CAD build for the part. Positions are in the model's coordinates, mm. Face numbers are marked on the shaded views. A direction names the side the tool comes from. Coordinates: 2 decimals unless noted, no trailing zeros. Loops run counter-clockwise (first coordinate to the right, second up) from the corner with the lowest first, then second, coordinate; pieces in that order, holes last. Notation, with made-up numbers: (31.25, 58.5) -> (59.25, 58.5) arc R22 cw to (59.25, 67.5) -> close; hole circle Ø4 at (-12, 54). An arc over 180 degrees is marked (long way). Return JSON: item names as keys, results as strings. Group by question number.
(1) Tool access for the marked faces 1, 2, 3, 4 and 5: list every direction of +Z, -Z, +X, -X, +Y, -Y with a clear straight run to the whole face (end or side of a thin tool).
(2) Flat gauge pins, fed straight in: pin 1 Ø2.5 at (x, y) = (16.5, 3.5) entering from -Z; pin 2 Ø1.8 at (x, z) = (-16, 17.5) entering from +Y; pin 3 Ø1.5 at (x, z) = (10.5, 27.5) entering from +Y; pin 4 Ø8 at (x, z) = (-12.5, 20.5) entering from +Y. Where does each tip first touch, or does it go through?
(3) Saw through at A-A on x = -1. Write the cut outline in (y, z), then the cut area to 3 significant figures.
(4) Probe L1, parallel to X at y = 5, z = 9.5; L2, parallel to X at y = -1.5, z = 29.5; L3, parallel to Y at x = -1.5, z = 15. List the from-to ranges inside material, lowest first.
(5) Saw through at B-B on y = 2.25. Write the cut outline in (x, z), then the cut area to 3 significant figures.
(6) Mould opens along Z. For the marked faces 6, 7 and 8 say: pulls with the +Z half, pulls with the -Z half, needs draft (parallel to the pull), parting line crosses it, or undercut.
(7) Saw through at C-C on z = 0.5. Write the cut outline in (x, y), then the cut area to 3 significant figures.
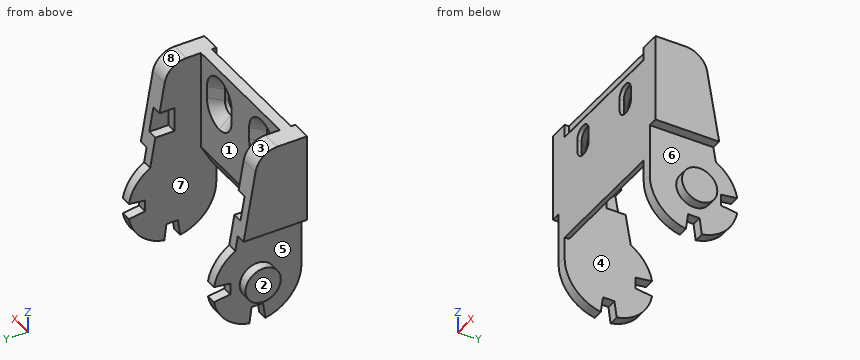
```python
from build123d import *

# Parameters (mm, degrees)
BODY_DEPTH                                       = 32
BODY_DEPTH_BACK                                  = 15
PIVOT_START                                      = 15
PIVOT_PIN_R_SKETCH_R                             = 4
PIVOT_PIN_R_DEPTH                                = 4.25
OUTSIDE_SHAPE_CUT_OUT_DEPTH                      = 40.272286666
OUTSIDE_SHAPE_CUT_OUT_DEPTH_BACK                 = 40.272286666
OUTSIDE_SHAPE_CUT_OUT_SKETCH_W                   = 49
OUTSIDE_SHAPE_CUT_OUT_SKETCH_H                   = 22
OUTSIDE_START                                    = 17.3
OUTSIDE_SHAPE_CUT_OUT_SKETCH_R_W                 = 24
OUTSIDE_SHAPE_CUT_OUT_SKETCH_R_H                 = 24
OUTSIDE_SHAPE_CUT_OUT_SKETCH_R_R                 = 4
OUTSIDE_SHAPE_CUT_OUT_R_DEPTH                    = 22.923727913
INSIDE_START                                     = 15
INSIDE_SHAPE_CUT_OUT_DEPTH                       = 30
LIGHTENING_START                                 = 1.25
LIGHTENING_2_SKETCH_W                            = 34.6
LIGHTENING_2_SKETCH_H                            = 5.5
LIGHTENING_2_DEPTH                               = 38.973727913
F_2_START                                        = -8.25
F_2_LATERAL_SLOTS_ORIENTATED_LONGITUDINALL_DEPTH = 3.5


with BuildPart() as part:
    # Profile Sketch → Body (new, two sides: drawn at the far end of the back side and taken through both)
    with BuildSketch(Plane.XY.offset(-BODY_DEPTH_BACK)):
        Polygon((-19.5, -8.25), (19.5, -8.25), (19.5, 11.75), (15, 11.75), (15, -4.75), (-15, -4.75), (-15, 11.75), (-19.5, 11.75), align=None)
    extrude(amount=BODY_DEPTH + BODY_DEPTH_BACK)

    # Pivot Pin R Sketch → Pivot Pin R (add)
    with BuildSketch(Plane(origin=(0, 0, 0), x_dir=(0, 0, -1), z_dir=(1, 0, 0)).offset(PIVOT_START)):
        with Locations((0, 1.75)):
            Circle(PIVOT_PIN_R_SKETCH_R)
    pivot_pin_r = extrude(amount=PIVOT_PIN_R_DEPTH)

    # Pivot Pin L: Pivot Pin R across plane
    add(pivot_pin_r.mirror(Plane(origin=(0, 0, 0), x_dir=(0, 0, 1), z_dir=(1, 0, 0))))

    # Outside Shape Cut Out Sketch → Outside Shape Cut Out (cut, two sides: drawn at the far end of the back side and taken through both)
    with BuildSketch(Plane(origin=(0, 0, 0), x_dir=(0, 0, -1), z_dir=(1, 0, 0)).offset(-OUTSIDE_SHAPE_CUT_OUT_DEPTH_BACK)):
        with Locations((-9.5, 0.75)):
            Rectangle(OUTSIDE_SHAPE_CUT_OUT_SKETCH_W, OUTSIDE_SHAPE_CUT_OUT_SKETCH_H)
        with BuildLine():
            Line((-27.844593584, 3.462159665), (-8.660254038, 6.75))
            ThreePointArc((-8.660254038, 6.75), (-5.762166553, 9.922969878), (-1.8, 11.586666102))
            Line((-1.8, 11.586666102), (-1.3, 7.87535696))
            Line((-1.3, 7.87535696), (1.3, 7.87535696))
            Line((1.3, 7.87535696), (1.8, 11.586666102))
            ThreePointArc((1.8, 11.586666102), (7.071067812, 8.821067812), (9.836666102, 3.55))
            Line((9.836666102, 3.55), (6.12535696, 3.05))
            Line((6.12535696, 3.05), (6.12535696, 0.45))
            Line((6.12535696, 0.45), (9.836666102, -0.05))
            ThreePointArc((9.836666102, -0.05), (6.403124237, -5.931145748), (0, -8.25))
            Line((0, -8.25), (-32, -8.25))
            Line((-32, -8.25), (-32, -1.46599026))
            ThreePointArc((-32, -1.46599026), (-30.822497084, 1.757131835), (-27.844593584, 3.462159665))
        make_face(mode=Mode.SUBTRACT)
    extrude(amount=OUTSIDE_SHAPE_CUT_OUT_DEPTH + OUTSIDE_SHAPE_CUT_OUT_DEPTH_BACK, mode=Mode.SUBTRACT)

    # Outside Shape Cut Out Sketch R → Outside Shape Cut Out R (cut, through all)
    with BuildSketch(Plane(origin=(0, 0, 0), x_dir=(0, 0, -1), z_dir=(1, 0, 0)).offset(OUTSIDE_START)):
        with Locations((0, 1.75)):
            Rectangle(OUTSIDE_SHAPE_CUT_OUT_SKETCH_R_W, OUTSIDE_SHAPE_CUT_OUT_SKETCH_R_H)
        with Locations((0, 1.75)):
            Circle(OUTSIDE_SHAPE_CUT_OUT_SKETCH_R_R, mode=Mode.SUBTRACT)
    outside_shape_cut_out_r = extrude(amount=OUTSIDE_SHAPE_CUT_OUT_R_DEPTH, mode=Mode.SUBTRACT)

    # Outside Shape Cut Out L: Outside Shape Cut Out R across plane
    add(outside_shape_cut_out_r.mirror(Plane(origin=(0, 0, 0), x_dir=(0, 0, 1), z_dir=(1, 0, 0))), mode=Mode.SUBTRACT)

    # Inside Shape Cut Out Sketch → Inside Shape Cut Out (cut)
    with BuildSketch(Plane(origin=(0, 0, 0), x_dir=(0, 0, -1), z_dir=(1, 0, 0)).offset(INSIDE_START)):
        Polygon((-29, -6.25), (-29, -8.25), (-32, -8.25), (-32, -7.25), (-30.5, -7.25), (-30.5, -6.25), align=None)
        Polygon((-9.5, -4.75), (-5, -7.25), (-5, -8.25), (7.599342077, -8.25), (7.599342077, -4.75), align=None)
    extrude(amount=-INSIDE_SHAPE_CUT_OUT_DEPTH, mode=Mode.SUBTRACT)

    # Lightening 2 Sketch → Lightening 2 (cut, through all)
    with BuildSketch(Plane(origin=(0, 0, 0), x_dir=(1, 0, 0), z_dir=(0, 1, 0)).offset(LIGHTENING_START)):
        with Locations((0, -18.25)):
            Rectangle(LIGHTENING_2_SKETCH_W, LIGHTENING_2_SKETCH_H)
    extrude(amount=LIGHTENING_2_DEPTH, mode=Mode.SUBTRACT)

    # 2 Lateral Slots Orientated Longitudinall: read off the stored shape, not the designer's step
    # 2 Lateral Slots Orientated Longitudi 2 → 2 Lateral Slots Orientated Longitudinall (cut)
    with BuildSketch(Plane(origin=(0, 0, 0), x_dir=(1, 0, 0), z_dir=(0, 1, 0)).offset(F_2_START)):
        with BuildLine():
            Line((5.85, -22.65), (5.85, -25.35))
            ThreePointArc((5.85, -25.35), (8, -27.5), (10.15, -25.35))
            Line((10.15, -25.35), (10.15, -22.65))
            ThreePointArc((10.15, -22.65), (8, -20.5), (5.85, -22.65))
        make_face()
        with BuildLine():
            Line((-10.15, -22.65), (-10.15, -25.35))
            ThreePointArc((-10.15, -25.35), (-8, -27.5), (-5.85, -25.35))
            Line((-5.85, -25.35), (-5.85, -22.65))
            ThreePointArc((-5.85, -22.65), (-8, -20.5), (-10.15, -22.65))
        make_face()
    extrude(amount=F_2_LATERAL_SLOTS_ORIENTATED_LONGITUDINALL_DEPTH, mode=Mode.SUBTRACT)

    # 2 Lateral Slots Orientated Longitudi 3: loft between two sections, ruled curve by curve
    f_2_lateral_slots_orientated_longitudi_3_from = [
        Edge.make_three_point_arc((5.85, -7.3, 25.35), (6.47972042, -7.3, 26.87027958), (8, -7.3, 27.5)),
        Edge.make_three_point_arc((8, -7.3, 27.5), (9.52027958, -7.3, 26.87027958), (10.15, -7.3, 25.35)),
        Edge.make_three_point_arc((10.15, -7.3, 22.65), (9.52027958, -7.3, 21.12972042), (8, -7.3, 20.5)),
        Edge.make_three_point_arc((8, -7.3, 20.5), (6.47972042, -7.3, 21.12972042), (5.85, -7.3, 22.65)),
        Edge.make_line((10.15, -7.3, 25.35), (10.15, -7.3, 22.65)),
        Edge.make_line((5.85, -7.3, 25.35), (5.85, -7.3, 22.65)),
    ]
    f_2_lateral_slots_orientated_longitudi_3_to = [
        Edge.make_three_point_arc((3.3, -4.75, 25.35), (4.676598128, -4.75, 28.673401872), (8, -4.75, 30.05)),
        Edge.make_three_point_arc((8, -4.75, 30.05), (11.323401872, -4.75, 28.673401872), (12.7, -4.75, 25.35)),
        Edge.make_three_point_arc((12.7, -4.75, 22.65), (11.323401872, -4.75, 19.326598128), (8, -4.75, 17.95)),
        Edge.make_three_point_arc((8, -4.75, 17.95), (4.676598128, -4.75, 19.326598128), (3.3, -4.75, 22.65)),
        Edge.make_line((12.7, -4.75, 25.35), (12.7, -4.75, 22.65)),
        Edge.make_line((3.3, -4.75, 25.35), (3.3, -4.75, 22.65)),
    ]
    f_2_lateral_slots_orientated_longitudi_3 = Solid(Shell([*[Face.make_surface_from_curves(f_2_lateral_slots_orientated_longitudi_3_from[k], f_2_lateral_slots_orientated_longitudi_3_to[k]) for k in range(6)], Face(Wire(f_2_lateral_slots_orientated_longitudi_3_from)), Face(Wire(f_2_lateral_slots_orientated_longitudi_3_to))]))
    add(f_2_lateral_slots_orientated_longitudi_3, mode=Mode.SUBTRACT)

    # 2 Lateral Slots Orientated Longitudi 4: loft between two sections, ruled curve by curve
    f_2_lateral_slots_orientated_longitudi_4_from = [
        Edge.make_three_point_arc((-10.15, -7.3, 25.35), (-9.52027958, -7.3, 26.87027958), (-8, -7.3, 27.5)),
        Edge.make_three_point_arc((-8, -7.3, 27.5), (-6.47972042, -7.3, 26.87027958), (-5.85, -7.3, 25.35)),
        Edge.make_three_point_arc((-5.85, -7.3, 22.65), (-6.47972042, -7.3, 21.12972042), (-8, -7.3, 20.5)),
        Edge.make_three_point_arc((-8, -7.3, 20.5), (-9.52027958, -7.3, 21.12972042), (-10.15, -7.3, 22.65)),
        Edge.make_line((-5.85, -7.3, 25.35), (-5.85, -7.3, 22.65)),
        Edge.make_line((-10.15, -7.3, 25.35), (-10.15, -7.3, 22.65)),
    ]
    f_2_lateral_slots_orientated_longitudi_4_to = [
        Edge.make_three_point_arc((-12.7, -4.75, 25.35), (-11.323401872, -4.75, 28.673401872), (-8, -4.75, 30.05)),
        Edge.make_three_point_arc((-8, -4.75, 30.05), (-4.676598128, -4.75, 28.673401872), (-3.3, -4.75, 25.35)),
        Edge.make_three_point_arc((-3.3, -4.75, 22.65), (-4.676598128, -4.75, 19.326598128), (-8, -4.75, 17.95)),
        Edge.make_three_point_arc((-8, -4.75, 17.95), (-11.323401872, -4.75, 19.326598128), (-12.7, -4.75, 22.65)),
        Edge.make_line((-3.3, -4.75, 25.35), (-3.3, -4.75, 22.65)),
        Edge.make_line((-12.7, -4.75, 25.35), (-12.7, -4.75, 22.65)),
    ]
    f_2_lateral_slots_orientated_longitudi_4 = Solid(Shell([*[Face.make_surface_from_curves(f_2_lateral_slots_orientated_longitudi_4_from[k], f_2_lateral_slots_orientated_longitudi_4_to[k]) for k in range(6)], Face(Wire(f_2_lateral_slots_orientated_longitudi_4_from)), Face(Wire(f_2_lateral_slots_orientated_longitudi_4_to))]))
    add(f_2_lateral_slots_orientated_longitudi_4, mode=Mode.SUBTRACT)


solid = part.part
```
Geometry results:
{
 "1": {"face 1": "+Z, -Z, +Y", "face 2": "+Z, -Z, -X, +Y, -Y", "face 3": "+Z, +X, -X, +Y", "face 4": "-Z, +Y", "face 5": "-X"},
 "2": {"pin 1": "z = -9.84", "pin 2": "y = 1.25", "pin 3": "y = -5.4", "pin 4": "y = 4.64"},
 "3": {"outline": "(-8.25, 5) -> (-7.25, 5) -> (-4.75, 9.5) -> (-4.75, 32) -> (-7.25, 32) -> (-7.25, 30.5) -> (-6.25, 30.5) -> (-6.25, 29) -> (-8.25, 29) -> close", "area": "84.4 mm²"},
 "4": {"L1": "-17.3 to -15, 15 to 17.3", "L2": "-19.5 to -15, 15 to 19.5", "L3": "-8.25 to -4.75"},
 "5": {"outline": "(-19.5, -3.97) -> (-17.3, -3.97) -> (-17.3, -6.13) -> (-15, -6.13) -> (-15, 15.5) -> (-17.3, 15.5) -> (-17.3, 21) -> (-15, 21) -> (-15, 30.35) -> (-19.5, 30.35) -> (-19.5, 12) -> (-17.3, 12) -> (-17.3, 3.97) -> (-19.5, 3.97) -> close; (15, -6.13) -> (17.3, -6.13) -> (17.3, -3.97) -> (19.5, -3.97) -> (19.5, 3.97) -> (17.3, 3.97) -> (17.3, 12) -> (19.5, 12) -> (19.5, 30.35) -> (15, 30.35) -> (15, 21) -> (17.3, 21) -> (17.3, 15.5) -> (15, 15.5) -> close", "area": "258 mm²"},
 "6": {"face 6": "undercut", "face 7": "needs draft", "face 8": "pulls with the +Z half"},
 "7": {"outline": "(-19.5, -2.22) -> (-17.3, -2.22) -> (-17.3, -8.25) -> (-15, -8.25) -> (-15, 7.88) -> (-17.3, 7.88) -> (-17.3, 5.72) -> (-19.5, 5.72) -> close; (15, -8.25) -> (17.3, -8.25) -> (17.3, -2.22) -> (19.5, -2.22) -> (19.5, 5.72) -> (17.3, 5.72) -> (17.3, 7.88) -> (15, 7.88) -> close", "area": "109 mm²"}
}
